from build123d import *

# Parameters (mm, degrees)
ESQUISSE1_W             = 70
ESQUISSE1_H             = 135
ESQUISSE1_R             = 1.25
BOSS_EXTRU_1_DEPTH      = 6
ENL_V_MAT_EXTRU_2_DEPTH = 153.187384497
ENL_V_MAT_EXTRU_3_DEPTH = 153.187384497


with BuildPart() as part:
    # Esquisse1 → Boss.-Extru.1 (new body)
    with BuildSketch(Plane.XY):
        with Locations((35, 67.5)):
            Rectangle(ESQUISSE1_W, ESQUISSE1_H)
        with Locations((62, 5)):
            Circle(ESQUISSE1_R, mode=Mode.SUBTRACT)
        with Locations((62, 15)):
            Circle(ESQUISSE1_R, mode=Mode.SUBTRACT)
        with Locations(Location((62, 120, 0), (0, 0, 180))):
            Circle(ESQUISSE1_R, mode=Mode.SUBTRACT)
        with Locations(Location((62, 130, 0), (0, 0, 180))):
            Circle(ESQUISSE1_R, mode=Mode.SUBTRACT)
    extrude(amount=BOSS_EXTRU_1_DEPTH)

    # Esquisse3 → Enlèv. mat.-Extru.2 (cut, through all)
    with BuildSketch(Plane.XY.offset(6)):
        with BuildLine():
            Line((70, 25.080128411), (70, 113.33030278))
            Line((70, 113.33030278), (55, 113.33030278))
            Line((55, 113.33030278), (55, 68.33030278))
            ThreePointArc((55, 68.33030278), (48.380211776, 41.80819896), (70, 25.080128411))
        make_face()
    extrude(amount=-ENL_V_MAT_EXTRU_2_DEPTH, mode=Mode.SUBTRACT)

    # Esquisse4 → Enlèv. mat.-Extru.3 (cut, through all)
    with BuildSketch(Plane(origin=(0, 0, 0), x_dir=(-1, 0, 0), z_dir=(0, 0, -1))):
        with BuildLine():
            Line((-12.9, 129), (-12.9, 121))
            ThreePointArc((-12.9, 121), (-14.5, 119.4), (-16.1, 121))
            Line((-16.1, 121), (-16.1, 129))
            ThreePointArc((-16.1, 129), (-14.5, 130.6), (-12.9, 129))
        make_face()
        with BuildLine():
            Line((-11.9, 89.5), (-11.9, 81.5))
            ThreePointArc((-11.9, 81.5), (-13.5, 79.9), (-15.1, 81.5))
            Line((-15.1, 81.5), (-15.1, 89.5))
            ThreePointArc((-15.1, 89.5), (-13.5, 91.1), (-11.9, 89.5))
        make_face()
        with BuildLine():
            Line((-30.9, 88.5), (-30.9, 80.5))
            ThreePointArc((-30.9, 80.5), (-32.5, 78.9), (-34.1, 80.5))
            Line((-34.1, 80.5), (-34.1, 88.5))
            ThreePointArc((-34.1, 88.5), (-32.5, 90.1), (-30.9, 88.5))
        make_face()
    extrude(amount=-ENL_V_MAT_EXTRU_3_DEPTH, mode=Mode.SUBTRACT)


solid = part.part
Work out the finished part from the listing and answer in its coordinate system (mm). A direction names the side the tool comes from. Give positions to 0.01 mm unless a question says otherwise; leave off trailing zeros. Order: outer loops, then holes, each group sorted by start corner. A loop starts at its lowest first (then second) coordinate and runs counter-clockwise, first axis right, second up. Notation, with made-up numbers: (89, 28) -> (142, 28) arc R29 cw to (142, 63) -> close; hole circle Ø1 at (0.5, -5). An arc over 180 degrees is marked (long way). Answer as a JSON object with one key per item and string values. Group by question number.
1. A flat-ended cylindrical pin translates along its axis: pin 1 Ø3 at (y, z) = (84.5, 3.5) entering from +X. Find the tip coordinate at first contact, or state that the pin passes through.
2. Section B-B on y = 86.5 is taken. Determine the outline of the cut face in (x, z), plus the area to 3 significant figures.
3. Section A-A on x = 32.5 is taken. Determine the outline of the cut face in (y, z), plus the area to 3 significant figures.
4. Consider line 1 along X through (y, z) = (85.5, 5.1); line 2 along X through (y, z) = (127, 3.85); line 3 along Y through (x, z) = (62, 4.4). Determine where each line is inside the solid, lowest interval first. Write a range as [from, to].
5. Section C-C on z = 4.1 is taken. Determine the outline of the cut face in (x, y).
6. Section D-D on y = 15 is taken. Determine the outline of the cut face in (x, z).
7. A tool of negligible diameter and unlimited length cuts with its end or side. For faces 1 (the flat face through (63, 113.33, 3)), 2 (the cylindrical face through (13.5, 91.1, 3)), 3 (the flat face through (70, 124, 3)), from which of +Z, -Z, +X, -X, +Y, -Y can it reach the whole face along a straight path? Write none if from no direction.
8. The mould has two halves that part along Y. Classify faces 4 (the cylindrical face through (48.25, 42.19, 3.04)), 5 (the flat face through (70, 12, 3)): released by +Y, released by -Y, zero draft, split by the parting line, or undercut.
Result sheet:
{
 "1": {"pin 1": "stops at x = 55"},
 "2": {"outline": "(0, 0) -> (11.9, 0) -> (11.9, 6) -> (0, 6) -> close; (15.1, 0) -> (30.9, 0) -> (30.9, 6) -> (15.1, 6) -> close; (34.1, 0) -> (55, 0) -> (55, 6) -> (34.1, 6) -> close", "area": "292 mm^2"},
 "3": {"outline": "(0, 0) -> (78.9, 0) -> (78.9, 6) -> (0, 6) -> close; (90.1, 0) -> (135, 0) -> (135, 6) -> (90.1, 6) -> close", "area": "743 mm^2"},
 "4": {"line 1": "x = [0, 11.9], [15.1, 30.9], [34.1, 55]", "line 2": "x = [0, 12.9], [16.1, 70]", "line 3": "y = [0, 3.75], [6.25, 13.75], [16.25, 27.09], [113.33, 118.75], [121.25, 128.75], [131.25, 135]"},
 "5": {"outline": "(0, 0) -> (70, 0) -> (70, 25.08) arc R25 cw to (55, 68.33) -> (55, 113.33) -> (70, 113.33) -> (70, 135) -> (0, 135) -> close; hole (11.9, 81.5) arc R1.6 ccw to (15.1, 81.5) -> (15.1, 89.5) arc R1.6 ccw to (11.9, 89.5) -> close; hole (12.9, 121) arc R1.6 ccw to (16.1, 121) -> (16.1, 129) arc R1.6 ccw to (12.9, 129) -> close; hole (30.9, 80.5) arc R1.6 ccw to (34.1, 80.5) -> (34.1, 88.5) arc R1.6 ccw to (30.9, 88.5) -> close; hole circle Ø2.5 at (62, 5); hole circle Ø2.5 at (62, 15); hole circle Ø2.5 at (62, 120); hole circle Ø2.5 at (62, 130)"},
 "6": {"outline": "(0, 0) -> (60.75, 0) -> (60.75, 6) -> (0, 6) -> close; (63.25, 0) -> (70, 0) -> (70, 6) -> (63.25, 6) -> close"},
 "7": {"face 1": "+Z, -Z, +X", "face 2": "+Z, -Z", "face 3": "+Z, -Z, +X, +Y, -Y"},
 "8": {"face 4": "undercut", "face 5": "zero draft"}
}
